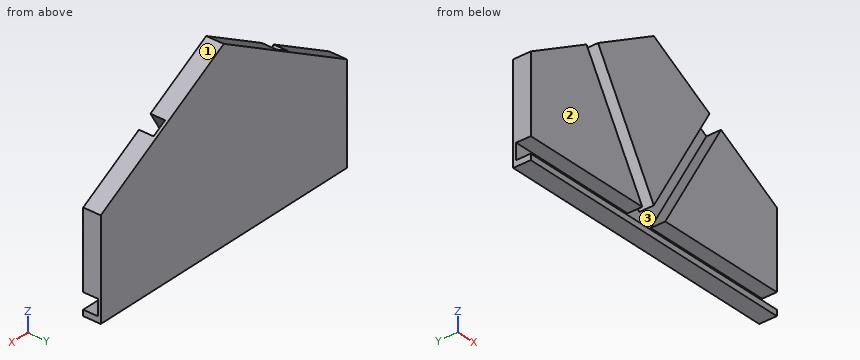
from build123d import *

# Parameters (mm, degrees)
BOSS_EXTRUDE1_DEPTH     = 6
SKETCH2_W               = 100
SKETCH2_H               = 5.4
CUT_EXTRUDE_THIN1_DEPTH = 5
SKETCH3_OUTSIDE_W       = 132.574
SKETCH3_OUTSIDE_H       = 148.044
CUT_EXTRUDE1_DEPTH      = 6


with BuildPart() as part:
    # Sketch1 → Boss-Extrude1 (new body)
    with BuildSketch(Plane(origin=(0, 0, 0), x_dir=(1, 0, 0), z_dir=(0, 1, 0))):
        Polygon((0, 57.735026919), (-50, 28.867513459), (-50, -28.867513459), (0, -57.735026919), (50, -28.867513459), (50, 28.867513459), align=None)
    extrude(amount=BOSS_EXTRUDE1_DEPTH)

    # Sketch2 → Cut-Extrude-Thin1 (cut)
    with BuildSketch(Plane.XZ):
        Polygon((-27.33826859, 41.951270189), (-3.33826859, 0.382050808), (1.33826859, 3.082050808), (-22.66173141, 44.651270189), align=None)
        Rectangle(SKETCH2_W, SKETCH2_H)
        Polygon((22.66173141, 44.651270189), (-1.33826859, 3.082050808), (3.33826859, 0.382050808), (27.33826859, 41.951270189), align=None)
    extrude(amount=-CUT_EXTRUDE_THIN1_DEPTH, mode=Mode.SUBTRACT)

    # Sketch3 outside → Cut-Extrude1 (cut)
    with BuildSketch(Plane.XZ):
        Rectangle(SKETCH3_OUTSIDE_W, SKETCH3_OUTSIDE_H)
        Polygon((-50, 28.867513459), (0, 57.735026919), (50, 28.867513459), (50, -4.7), (-50, -4.7), align=None, mode=Mode.SUBTRACT)
    extrude(amount=-CUT_EXTRUDE1_DEPTH, mode=Mode.SUBTRACT)


solid = part.part
Work out the finished part from the listing and answer in its coordinate system (mm). Face numbers are marked on the shaded views. Give positions to 0.01 mm unless a question says otherwise; leave off trailing zeros. Loops run counter-clockwise (first coordinate to the right, second up) from the corner with the lowest first, then second, coordinate; pieces in that order, holes last. Notation, with made-up numbers: (9, 19.5) - (43, 19.5) arc R12 cw to (43, 32.5) - close; hole circle Ø7 at (68, 15.25). An arc over 180 degrees is marked (long way). Answer in a Markdown table with one row per item. Add a question column.
Q1. The part is cut by section B-B (z = 30.5). Determine the outline of the cut face in (x, y).
Q2. The part is cut by section C-C (x = -15.5). Determine the outline of the cut face in (y, z).
Q3. Consider line 1 along Z through (x, y) = (9, 3.55); line 2 along Z through (x, y) = (7, 1.2); line 3 along X through (y, z) = (4.5, 13.5). Determine where each line is inside the solid, lowest interval first.
Q4. The part is cut by section D-D (z = 0). Determine the outline of the cut face in (x, y), and give its area (3 significant figures).
Q5. Each of these flat-tipped pins is pushed along its axis until it touches: P1, Ø1.5, axis at x = 14, y = 2.5, coming from the +Z side; P2, Ø1.5, axis at x = 18, y = 3.5, coming from the +Z side; P3, Ø1, axis at y = 5, z = 39, coming from the -X side. Where does it stop, or does it pass through?
Q6. The part is cut by section A-A (y = 2.8). Determine the outline of the cut face in (x, z).
Q7. Determine the mould class of the marked faces 1, 2 and 3 for opening direction Z: released by +Z, released by -Z, zero draft, split by the parting line, or undercut.
Solution:
| question | item | result |
|---|---|---|
| 1 | outline | (-47.17, 0) - (-20.73, 0) - (-20.73, 5) - (-14.49, 5) - (-14.49, 0) - (14.49, 0) - (14.49, 5) - (20.73, 5) - (20.73, 0) - (47.17, 0) - (47.17, 6) - (-47.17, 6) - close |
| 2 | outline | (0, -4.7) - (6, -4.7) - (6, 48.79) - (0, 48.79) - (0, 32.25) - (5, 32.25) - (5, 21.45) - (0, 21.45) - (0, 2.7) - (5, 2.7) - (5, -2.7) - (0, -2.7) - close |
| 3 | line 1 | z = -4.7 to -2.7, 2.7 to 10.19, 20.99 to 52.54 |
| 3 | line 2 | z = -4.7 to -2.7, 2.7 to 6.72, 17.52 to 53.69 |
| 3 | line 3 | x = -50 to -10.91, -4.68 to 4.68, 10.91 to 50 |
| 4 | outline | (-50, 5) - (50, 5) - (50, 6) - (-50, 6) - close |
| 4 | area | 100 mm² |
| 5 | P1 | stops at z = 50.09 |
| 5 | P2 | stops at z = 47.78 |
| 5 | P3 | stops at x = -33.32 |
| 6 | outline | (-50, -4.7) - (50, -4.7) - (50, -2.7) - (-50, -2.7) - close; (-50, 2.7) - (-4.68, 2.7) - (-27.34, 41.95) - (-50, 28.87) - close; (-22.66, 44.65) - (0, 5.4) - (22.66, 44.65) - (0, 57.74) - close; (4.68, 2.7) - (50, 2.7) - (50, 28.87) - (27.34, 41.95) - close |
| 7 | face 1 | released by +Z |
| 7 | face 2 | zero draft |
| 7 | face 3 | undercut |
